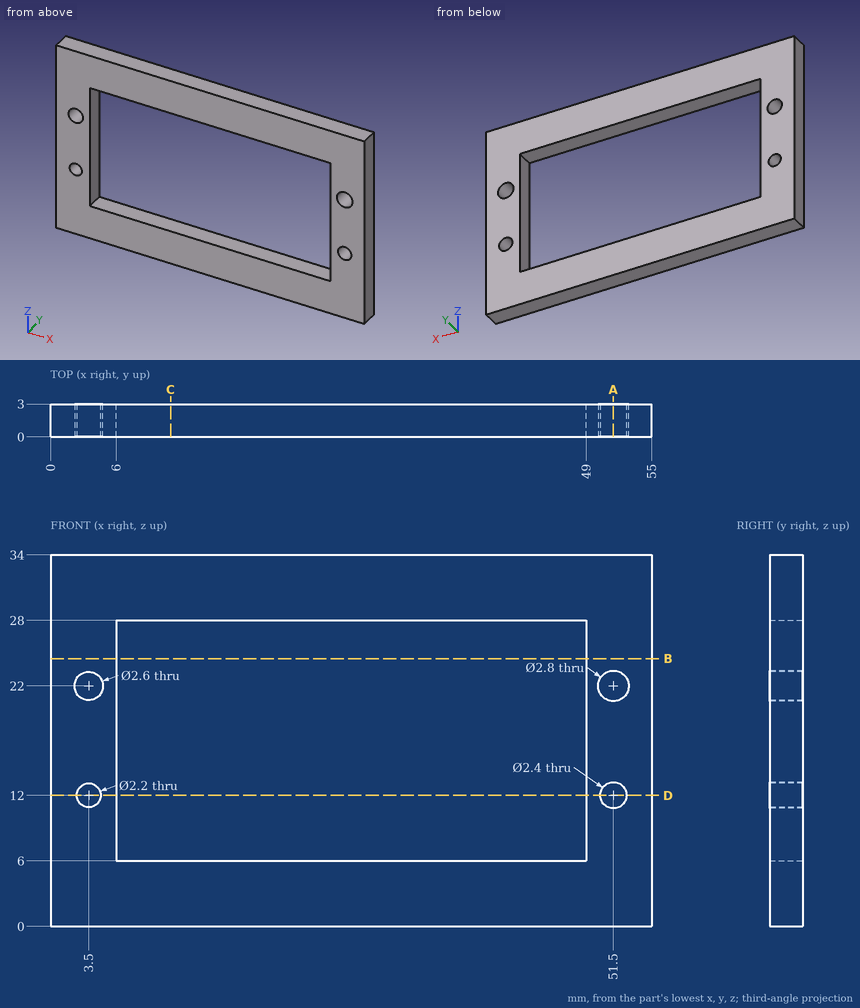
For this review, use the dimensioned drawing (mm, ordinates from the lowest corner) and the shaded views. Coordinates: 2 decimals unless noted, no trailing zeros. Loops run counter-clockwise (first coordinate to the right, second up) from the corner with the lowest first, then second, coordinate; pieces in that order, holes last. Notation, with made-up numbers: (-13, 59.25) -> (36, 59.25) arc R18 ccw to (36, 79.25) -> close; hole circle Ø7 at (-24.75, -26.5). An arc over 180 degrees is marked (long way). Return JSON: item names as keys, results as strings. Group by question number.
(1) Consider section C-C, the plane x = 11. Give the boundary of the cut face in (y, z).
(2) Consider section D-D, the plane z = 12. Give the boundary of the cut face in (x, y), plus the area to 3 significant figures.
(3) Consider section B-B, the plane z = 24.5. Give the boundary of the cut face in (x, y).
(4) To check wall thickness, follow L1, parallel to Z at x = 3.5, y = 0.8; L2, parallel to X at y = 2.05, z = 22; L3, parallel to X at y = 1.75, z = 12. State the ranges of each line that lie inside material, in increasing order.
(5) Consider section A-A, the plane x = 51.5. Give the boundary of the cut face in (y, z).
Results below:
{
 "1": {"outline": "(0, 0) -> (3, 0) -> (3, 6) -> (0, 6) -> close; (0, 28) -> (3, 28) -> (3, 34) -> (0, 34) -> close"},
 "2": {"outline": "(0, 0) -> (2.4, 0) -> (2.4, 3) -> (0, 3) -> close; (4.6, 0) -> (6, 0) -> (6, 3) -> (4.6, 3) -> close; (49, 0) -> (50.3, 0) -> (50.3, 3) -> (49, 3) -> close; (52.7, 0) -> (55, 0) -> (55, 3) -> (52.7, 3) -> close", "area": "22.2 mm2"},
 "3": {"outline": "(0, 0) -> (6, 0) -> (6, 3) -> (0, 3) -> close; (49, 0) -> (55, 0) -> (55, 3) -> (49, 3) -> close"},
 "4": {"L1": "z = 0 to 10.9, 13.1 to 20.7, 23.3 to 34", "L2": "x = 0 to 2.2, 4.8 to 6, 49 to 50.1, 52.9 to 55", "L3": "x = 0 to 2.4, 4.6 to 6, 49 to 50.3, 52.7 to 55"},
 "5": {"outline": "(0, 0) -> (3, 0) -> (3, 10.8) -> (0, 10.8) -> close; (0, 13.2) -> (3, 13.2) -> (3, 20.6) -> (0, 20.6) -> close; (0, 23.4) -> (3, 23.4) -> (3, 34) -> (0, 34) -> close"}
}
